Answer from the drawing. Dimensions are ordinates in mm from the lowest x, y and z of the part. Give positions to 0.01 mm unless a question says otherwise; leave off trailing zeros. Write each loop counter-clockwise with the first axis right and the second up, starting at its lowest first coordinate (ties: lowest second). Pieces come first, ordered by that corner, then holes.
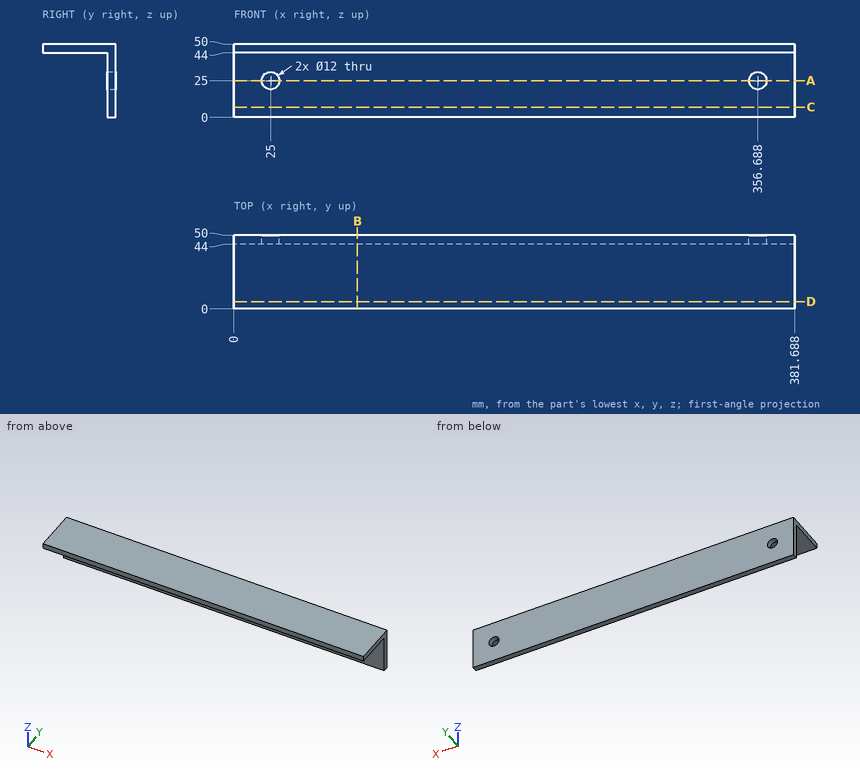
Item 1: Each of these flat-tipped pins is pushed along its axis until it touches: P1, Ø22, axis at x = 242.5, y = 25.5, coming from the -Z side; P2, Ø14, axis at x = 25, z = 25, coming from the -Y side. Where does it stop, or does it pass through?
Conclusion:
P1: stops at z = 44
P2: stops at y = 44
Item 2: Consider probe 1 along X at (y, z) = (47.05, 25); probe 2 along Y at (x, z) = (129.5, 40.5); probe 3 along Z at (x, y) = (25, 46). Determine where each line is inside the solid, lowest interval first.
Conclusion:
probe 1: x = 0 to 19, 31 to 350.69, 362.69 to 381.69
probe 2: y = 44 to 50
probe 3: z = 0 to 19, 31 to 50
Item 3: A cutting plane is placed at A-A, the plane z = 25. Give the vertices of the cut face in (x, y), plus the area to 3 significant figures.
Conclusion:
outline: (0, 44) - (19, 44) - (19, 50) - (0, 50) - close; (31, 44) - (350.69, 44) - (350.69, 50) - (31, 50) - close; (362.69, 44) - (381.69, 44) - (381.69, 50) - (362.69, 50) - close
area: 2,150 mm2
Item 4: A cutting plane is placed at B-B, the plane x = 84. Give the vertices of the cut face in (y, z), plus the area to 3 significant figures.
Conclusion:
outline: (0, 44) - (44, 44) - (44, 0) - (50, 0) - (50, 50) - (0, 50) - close
area: 564 mm2
Item 5: A cutting plane is placed at C-C, the plane z = 7. Give the vertices of the cut face in (x, y).
Conclusion:
outline: (0, 44) - (381.69, 44) - (381.69, 50) - (0, 50) - close
